Geometry: final body of the model. Coordinates: model frame, mm. Face numbers are marked on the shaded views. A direction names the side the tool comes from. Coordinates: 2 decimals unless noted, no trailing zeros. Write each loop counter-clockwise with the first axis right and the second up, starting at its lowest first coordinate (ties: lowest second). Pieces come first, ordered by that corner, then holes. Notation, with made-up numbers: (-37.5, 76.5) -> (-24.5, 76.5) arc R11 cw to (-24.5, 85.5) -> close; hole circle Ø5 at (32.25, 34). An arc over 180 degrees is marked (long way). Answer as a JSON object with one key per item and string values. Group by question number.
```python
from build123d import *

# Parameters (mm, degrees)
F0_R     = 17.4495
F1_DEPTH = 25
F2_R     = 26.49903
F2_R_2   = 15.5
F3_DEPTH = 15
F4_R     = 10
F5_DEPTH = 28


with BuildPart() as f1:
    # F0 (on Front) → F1 (new body)
    with BuildSketch(Plane.XZ):
        Circle(F0_R)
    extrude(amount=F1_DEPTH)

    # F2 (on face) → F3 (cut)
    with BuildSketch(Plane(origin=(0, 0, 0), x_dir=(-1, 0, 0), z_dir=(0, 1, 0))):
        with Locations((2.900601, 0)):
            Circle(F2_R)
        Circle(F2_R_2, mode=Mode.SUBTRACT)
    extrude(amount=-F3_DEPTH, mode=Mode.SUBTRACT)

    # F4 (on face) → F5 (join)
    with BuildSketch(Plane(origin=(0, 0, 0), x_dir=(-1, 0, 0), z_dir=(0, 1, 0))):
        Circle(F4_R)
    extrude(amount=F5_DEPTH)


solid = f1.part
```
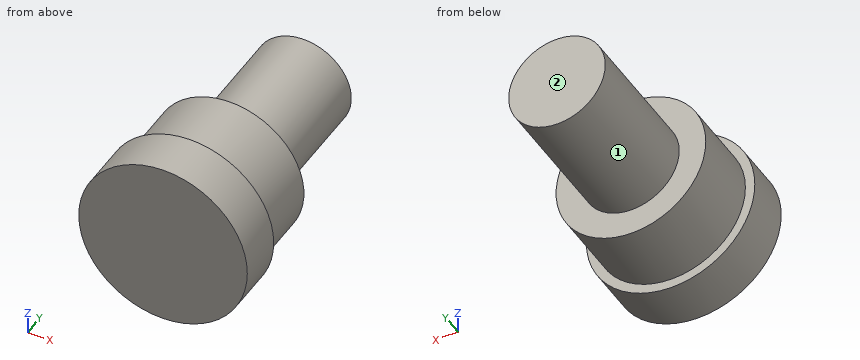
Item 1: Section B-B on x = 0. Output: boundary loops of the cut face in (y, z).
Item 2: Section A-A on z = 0. Output: boundary loops of the cut face in (x, y).
Item 3: Section D-D on y = -9. Output: boundary loops of the cut face in (x, z), then the cut area to 3 significant figures.
Item 4: Ray query, L1, parallel to Y at x = -12.5, z = 4.5; L2, parallel to Z at x = -0.5, y = 23.5; L3, parallel to X at y = -8, z = -13. Return the intervals inside material, ascending. Write a range as [from, to].
Item 5: Section C-C on y = 4. Output: boundary loops of the cut face in (x, z).
Item 6: Contact query for flat-ended pins moving along their axis: pin 1 (4 mm diameter, centred on x = -5.5, y = -16, fed in from +Z); pin 2 (2 mm diameter, centred on y = 21.5, z = 9, fed in from +X); pin 3 (1 mm diameter, centred on x = 9.5, y = 15, fed in from -Z). Output: stop coordinate, or through.
Item 7: Set-up query: the marked faces 1 and 2. Return all of +Z, -Z, +X, -X, +Y, -Y with unobstructed straight access to the full face (end or side cutting, diameter ignored); none if empty.
Answer sheet:
{
 "1": {"outline": "(-25, -17.45) -> (-15, -17.45) -> (-15, -15.5) -> (0, -15.5) -> (0, -10) -> (28, -10) -> (28, 10) -> (0, 10) -> (0, 15.5) -> (-15, 15.5) -> (-15, 17.45) -> (-25, 17.45) -> close"},
 "2": {"outline": "(-17.45, -25) -> (17.45, -25) -> (17.45, -15) -> (15.5, -15) -> (15.5, 0) -> (10, 0) -> (10, 28) -> (-10, 28) -> (-10, 0) -> (-15.5, 0) -> (-15.5, -15) -> (-17.45, -15) -> close"},
 "3": {"outline": "circle Ø31 at (0, 0)", "area": "755 mm^2"},
 "4": {"L1": "y = [-25, 0]", "L2": "z = [-9.99, 9.99]", "L3": "x = [-8.44, 8.44]"},
 "5": {"outline": "circle Ø20 at (0, 0)"},
 "6": {"pin 1": "stops at z = 17.09", "pin 2": "stops at x = 6", "pin 3": "stops at z = -4.36"},
 "7": {"face 1": "+Y", "face 2": "+Z, -Z, +X, -X, +Y"}
}
